The model under review builds one solid part; all positions refer to its coordinate system, in mm. A direction names the side the tool comes from. Round coordinates to 2 decimals unless told otherwise and drop trailing zeros. Loops run counter-clockwise (first coordinate to the right, second up) from the corner with the lowest first, then second, coordinate; pieces in that order, holes last. Notation, with made-up numbers: M 63.25,0 L 122.25,0 A8 cw 122.25,7 Z; hole C 57.25,2 d9. An arc over 180 degrees is marked long. Answer as a JSON object with one key per item and string values. Group by question number.
Item 1: The part is to be moulded in two halves that separate along X. For faces 1 (the face through (-54.1, -28.64, 0.99)), 2 (the face through (-1, 29, 2)), 3 (the face through (13.14, 84.6, 0.99)), 4 (the face through (-39.5, 67.4, 1)), say which applies: +X half, -X half, draft (parallel to the pull), parting line (faces both ways), or undercut.
Item 2: Consider section C-C (z = 1.45). State how many separate pieces and enclosed holes the cut face has, and give its area (3 significant figures).
Item 3: Consider section A-A (x = -3.5). Give the boundary of the cut face in (y, z).
Item 4: Consider section B-B (y = 58). Give the boundary of the cut face in (x, z), and give its area (3 significant figures).
Item 5: Insertion check: P1, Ø0.6, axis at y = 35.5, z = 1.5, coming from the -X side; P2, Ø3, axis at x = 38, y = 79, coming from the -Z side; P3, Ø1, axis at y = 80, z = 1, coming from the +X side. Each pin has a flat end and moves straight along its axis. Give the tip position at first contact, or say it passes through.
Item 6: Tool access review of faces 5 (the face through (-48.5, 67.6, 1)), 6 (the face through (-54.14, 31.6, 1.01)), 7 (the face through (24.14, 72.6, 0.99)): name each direction out of +Z, -Z, +X, -X, +Y, -Y from which nothing blocks a thin tool from reaching the whole face with its end or side.
Item 7: To check wall thickness, follow line 1 (Y direction, x = 0.75, z = 1.15); line 2 (X direction, y = 79, z = 1.8); line 3 (Y direction, x = -23.5, z = 1.85). State the ranges of each line that lie inside material, in increasing order.
```python
from build123d import *

# Parameters (mm, degrees)
SKETCH_1_W          = 110
SKETCH_1_H          = 65
EXTRUDE_1_DEPTH     = 2
FILLET_1_R          = 3
SKETCH_2_R          = 3
EXTRUDE_2_DEPTH     = 2
FILLET_5_R          = 3
FILLET_6_R          = 5
SKETCH_4_W          = 10
SKETCH_4_H          = 5
EXTRUDE_4_DEPTH     = 2
FILLET_7_R          = 0.5
SKETCH_5_W          = 16
SKETCH_5_H          = 45
SKETCH_5_R          = 1.2
EXTRUDE_5_DEPTH     = 2
SKETCH_6_W          = 10
SKETCH_6_H          = 5
SKETCH_6_W_2        = 5
SKETCH_6_H_2        = 10
EXTRUDE_6_DEPTH     = 2
FILLET_8_R          = 0.5
FILLET_9_R          = 2
SKETCH_7_W          = 110
SKETCH_7_H          = 3
CUT_EXTRUDE_1_DEPTH = 10
FILLET_10_R         = 3
SKETCH_10_W         = 5
SKETCH_10_H         = 19.84178834
CUT_EXTRUDE_3_DEPTH = 10
SKETCH_11_R         = 0.375
CUT_EXTRUDE_4_DEPTH = 10


with BuildPart() as part:
    # Sketch 1 → Extrude 1 (new body)
    with BuildSketch(Plane.XY):
        Rectangle(SKETCH_1_W, SKETCH_1_H)
        with BuildLine():
            Line((-49.5, 24.75), (-46.5, 24.75))
            ThreePointArc((-46.5, 24.75), (-44.75, 26.5), (-46.5, 28.25))
            Line((-46.5, 28.25), (-49.5, 28.25))
            ThreePointArc((-49.5, 28.25), (-51.25, 26.5), (-49.5, 24.75))
        make_face(mode=Mode.SUBTRACT)
        with BuildLine():
            Line((-46.5, -20.25), (-49.5, -20.25))
            ThreePointArc((-49.5, -20.25), (-51.25, -18.5), (-49.5, -16.75))
            Line((-49.5, -16.75), (-46.5, -16.75))
            ThreePointArc((-46.5, -16.75), (-44.75, -18.5), (-46.5, -20.25))
        make_face(mode=Mode.SUBTRACT)
        with BuildLine():
            Line((46.5, -20.25), (49.5, -20.25))
            ThreePointArc((49.5, -20.25), (51.25, -18.5), (49.5, -16.75))
            Line((49.5, -16.75), (46.5, -16.75))
            ThreePointArc((46.5, -16.75), (44.75, -18.5), (46.5, -20.25))
        make_face(mode=Mode.SUBTRACT)
        with BuildLine():
            Line((46.5, 28.25), (49.5, 28.25))
            ThreePointArc((49.5, 28.25), (51.25, 26.5), (49.5, 24.75))
            Line((49.5, 24.75), (46.5, 24.75))
            ThreePointArc((46.5, 24.75), (44.75, 26.5), (46.5, 28.25))
        make_face(mode=Mode.SUBTRACT)
    extrude(amount=EXTRUDE_1_DEPTH)

    # Fillet 1
    fillet_1_edges = [part.edges().sort_by_distance(p)[0] for p in [
        (-55, 32.5, 1),
        (55, 32.5, 1),
    ]]
    fillet(fillet_1_edges, radius=FILLET_1_R)



with BuildPart() as body_2:
    # Sketch 2 → Extrude 2 (new body)
    with BuildSketch(Plane.XY.offset(2)):
        Polygon((-55, 37.5), (25, 37.5), (25, 73.5), (14, 73.5), (14, 85.5), (-44, 85.5), (-44, 73.5), (-55, 73.5), align=None)
        with Locations((14, 67.5)):
            Circle(SKETCH_2_R, mode=Mode.SUBTRACT)
        with BuildLine():
            Line((-45.5, 64.5), (-42.5, 64.5))
            ThreePointArc((-42.5, 64.5), (-39.5, 67.5), (-42.5, 70.5))
            Line((-42.5, 70.5), (-45.5, 70.5))
            ThreePointArc((-45.5, 70.5), (-48.5, 67.5), (-45.5, 64.5))
        make_face(mode=Mode.SUBTRACT)
    extrude(amount=-EXTRUDE_2_DEPTH)

    # Fillet 5
    fillet_5_edges = [body_2.edges().sort_by_distance(p)[0] for p in [
        (25, 37.5, 1),
        (-55, 37.5, 1),
        (-55, 73.5, 1),
        (-44, 85.5, 1),
        (14, 85.5, 1),
        (25, 73.5, 1),
    ]]
    fillet(fillet_5_edges, radius=FILLET_5_R)

    # Fillet 6
    fillet_6_edges = [body_2.edges().sort_by_distance(p)[0] for p in [
        (-44, 73.5, 1),
        (14, 73.5, 1),
    ]]
    fillet(fillet_6_edges, radius=FILLET_6_R)


with BuildPart() as part_1:
    add(part.part)

    add(body_2.part)  # Extrude 4 merges body 2
    # Sketch 4 → Extrude 4 (add)
    with BuildSketch(Plane.XY.offset(2)):
        with Locations((-35, 35)):
            Rectangle(SKETCH_4_W, SKETCH_4_H)
        with Locations((5, 35)):
            Rectangle(SKETCH_4_W, SKETCH_4_H)
    extrude(amount=-EXTRUDE_4_DEPTH)

    # Fillet 7
    fillet_7_edges = [part_1.edges().sort_by_distance(p)[0] for p in [
        (0, 37.5, 1),
        (10, 37.5, 1),
        (10, 32.5, 1),
        (0, 32.5, 1),
        (-40, 37.5, 1),
        (-30, 37.5, 1),
        (-30, 32.5, 1),
        (-40, 32.5, 1),
    ]]
    fillet(fillet_7_edges, radius=FILLET_7_R)



with BuildPart() as body_2_2:
    # Sketch 5 → Extrude 5 (new body)
    with BuildSketch(Plane.XY.offset(2)):
        with Locations((38, 60)):
            Rectangle(SKETCH_5_W, SKETCH_5_H)
        with Locations((38, 79)):
            Circle(SKETCH_5_R, mode=Mode.SUBTRACT)
        with BuildLine():
            Line((36.683223365, 42), (36.683223365, 40))
            ThreePointArc((36.683223365, 40), (37.883223365, 38.8), (39.083223365, 40))
            Line((39.083223365, 40), (39.083223365, 42))
            ThreePointArc((39.083223365, 42), (37.883223365, 43.2), (36.683223365, 42))
        make_face(mode=Mode.SUBTRACT)
    extrude(amount=-EXTRUDE_5_DEPTH)


with BuildPart() as part_2:
    add(part_1.part)

    add(body_2_2.part)  # Extrude 6 merges body 2 2
    # Sketch 6 → Extrude 6 (add)
    with BuildSketch(Plane.XY.offset(2)):
        with Locations((38, 35)):
            Rectangle(SKETCH_6_W, SKETCH_6_H)
        with Locations((27.5, 60.5)):
            Rectangle(SKETCH_6_W_2, SKETCH_6_H_2)
    extrude(amount=-EXTRUDE_6_DEPTH)

    # Fillet 8
    fillet_8_edges = [part_2.edges().sort_by_distance(p)[0] for p in [
        (33, 37.5, 1),
        (43, 37.5, 1),
        (43, 32.5, 1),
        (33, 32.5, 1),
        (25, 55.5, 1),
        (25, 65.5, 1),
        (30, 65.5, 1),
        (30, 55.5, 1),
    ]]
    fillet(fillet_8_edges, radius=FILLET_8_R)

    # Fillet 9
    fillet_9_edges = [part_2.edges().sort_by_distance(p)[0] for p in [
        (46, 37.5, 1),
        (46, 82.5, 1),
        (30, 37.5, 1),
        (30, 82.5, 1),
    ]]
    fillet(fillet_9_edges, radius=FILLET_9_R)

    # Sketch 7 → Cut-Extrude 1 (cut)
    with BuildSketch(Plane.XY.offset(2)):
        with Locations((0, -31)):
            Rectangle(SKETCH_7_W, SKETCH_7_H)
    extrude(amount=-CUT_EXTRUDE_1_DEPTH, mode=Mode.SUBTRACT)

    # Fillet 10
    fillet_10_edges = [part_2.edges().sort_by_distance(p)[0] for p in [
        (55, -29.5, 1),
        (-55, -29.5, 1),
    ]]
    fillet(fillet_10_edges, radius=FILLET_10_R)

    # Sketch 10 → Cut-Extrude 3 (cut)
    with BuildSketch(Plane.XY.offset(2)):
        with Locations((27.5, 60.5)):
            Rectangle(SKETCH_10_W, SKETCH_10_H)
    extrude(amount=-CUT_EXTRUDE_3_DEPTH, mode=Mode.SUBTRACT)

    # Sketch 11 → Cut-Extrude 4 (cut)
    with BuildSketch(Plane.XY.offset(2)):
        with Locations((-39.25, 37.125)):
            Circle(SKETCH_11_R)
        with Locations((-38.05, 37.125)):
            Circle(SKETCH_11_R)
        with Locations((-36.85, 37.125)):
            Circle(SKETCH_11_R)
        with Locations((-35.65, 37.125)):
            Circle(SKETCH_11_R)
        with Locations((-34.45, 37.125)):
            Circle(SKETCH_11_R)
        with Locations((-33.25, 37.125)):
            Circle(SKETCH_11_R)
        with Locations((-32.05, 37.125)):
            Circle(SKETCH_11_R)
        with Locations((-30.85, 37.125)):
            Circle(SKETCH_11_R)
        with Locations((0.75, 37.125)):
            Circle(SKETCH_11_R)
        with Locations((33.75, 37.125)):
            Circle(SKETCH_11_R)
        with Locations((34.95, 37.125)):
            Circle(SKETCH_11_R)
        with Locations((36.15, 37.125)):
            Circle(SKETCH_11_R)
        with Locations((37.35, 37.125)):
            Circle(SKETCH_11_R)
        with Locations((38.55, 37.125)):
            Circle(SKETCH_11_R)
        with Locations((39.75, 37.125)):
            Circle(SKETCH_11_R)
        with Locations((40.95, 37.125)):
            Circle(SKETCH_11_R)
        with Locations((42.15, 37.125)):
            Circle(SKETCH_11_R)
        with Locations((1.95, 37.125)):
            Circle(SKETCH_11_R)
        with Locations((3.15, 37.125)):
            Circle(SKETCH_11_R)
        with Locations((4.35, 37.125)):
            Circle(SKETCH_11_R)
        with Locations((5.55, 37.125)):
            Circle(SKETCH_11_R)
        with Locations((6.75, 37.125)):
            Circle(SKETCH_11_R)
        with Locations((7.95, 37.125)):
            Circle(SKETCH_11_R)
        with Locations((9.15, 37.125)):
            Circle(SKETCH_11_R)
        with Locations(Location((42.15, 32.875, 0), (0, 0, 180))):
            Circle(SKETCH_11_R)
        with Locations(Location((40.95, 32.875, 0), (0, 0, 180))):
            Circle(SKETCH_11_R)
        with Locations(Location((39.75, 32.875, 0), (0, 0, 180))):
            Circle(SKETCH_11_R)
        with Locations(Location((38.55, 32.875, 0), (0, 0, 180))):
            Circle(SKETCH_11_R)
        with Locations(Location((37.35, 32.875, 0), (0, 0, 180))):
            Circle(SKETCH_11_R)
        with Locations(Location((36.15, 32.875, 0), (0, 0, 180))):
            Circle(SKETCH_11_R)
        with Locations(Location((34.95, 32.875, 0), (0, 0, 180))):
            Circle(SKETCH_11_R)
        with Locations(Location((33.75, 32.875, 0), (0, 0, 180))):
            Circle(SKETCH_11_R)
        with Locations(Location((0.75, 32.875, 0), (0, 0, 180))):
            Circle(SKETCH_11_R)
        with Locations(Location((1.95, 32.875, 0), (0, 0, 180))):
            Circle(SKETCH_11_R)
        with Locations(Location((3.15, 32.875, 0), (0, 0, 180))):
            Circle(SKETCH_11_R)
        with Locations(Location((4.35, 32.875, 0), (0, 0, 180))):
            Circle(SKETCH_11_R)
        with Locations(Location((5.55, 32.875, 0), (0, 0, 180))):
            Circle(SKETCH_11_R)
        with Locations(Location((6.75, 32.875, 0), (0, 0, 180))):
            Circle(SKETCH_11_R)
        with Locations(Location((7.95, 32.875, 0), (0, 0, 180))):
            Circle(SKETCH_11_R)
        with Locations(Location((9.15, 32.875, 0), (0, 0, 180))):
            Circle(SKETCH_11_R)
        with Locations(Location((-30.85, 32.875, 0), (0, 0, 180))):
            Circle(SKETCH_11_R)
        with Locations(Location((-32.05, 32.875, 0), (0, 0, 180))):
            Circle(SKETCH_11_R)
        with Locations(Location((-33.25, 32.875, 0), (0, 0, 180))):
            Circle(SKETCH_11_R)
        with Locations(Location((-34.45, 32.875, 0), (0, 0, 180))):
            Circle(SKETCH_11_R)
        with Locations(Location((-35.65, 32.875, 0), (0, 0, 180))):
            Circle(SKETCH_11_R)
        with Locations(Location((-36.85, 32.875, 0), (0, 0, 180))):
            Circle(SKETCH_11_R)
        with Locations(Location((-38.05, 32.875, 0), (0, 0, 180))):
            Circle(SKETCH_11_R)
        with Locations(Location((-39.25, 32.875, 0), (0, 0, 180))):
            Circle(SKETCH_11_R)
    extrude(amount=-CUT_EXTRUDE_4_DEPTH, mode=Mode.SUBTRACT)


solid = part_2.part
```
Geometry results:
{
 "1": {"face 1": "-X half", "face 2": "draft", "face 3": "+X half", "face 4": "undercut"},
 "2": {"separate pieces": "1", "enclosed holes": "57", "area": "11,100 mm^2"},
 "3": {"outline": "M -29.5,0 L 32.5,0 L 32.5,2 L -29.5,2 Z; M 37.5,0 L 85.5,0 L 85.5,2 L 37.5,2 Z"},
 "4": {"outline": "M -55,0 L 25,0 L 25,2 L -55,2 Z; M 30,0 L 46,0 L 46,2 L 30,2 Z", "area": "192 mm^2"},
 "5": {"P1": "stops at x = -40", "P2": "stops at z = 0", "P3": "stops at x = 46"},
 "6": {"face 5": "+Z, -Z", "face 6": "+Z, -Z, -X", "face 7": "+Z, -Z, +Y"},
 "7": {"line 1": "y = -29.5 to 32.5, 33.25 to 36.75, 37.5 to 85.5", "line 2": "x = -44 to 14, 30 to 36.8, 39.2 to 46", "line 3": "y = -29.5 to 32.5, 37.5 to 85.5"}
}
